Job drawing, mm, ordinate dimensions from the low corner. One solid piece. A direction names the side the tool comes from. Give positions to 0.01 mm unless a question says otherwise; leave off trailing zeros. Order: outer loops, then holes, each group sorted by start corner. A loop starts at its lowest first (then second) coordinate and runs counter-clockwise, first axis right, second up.
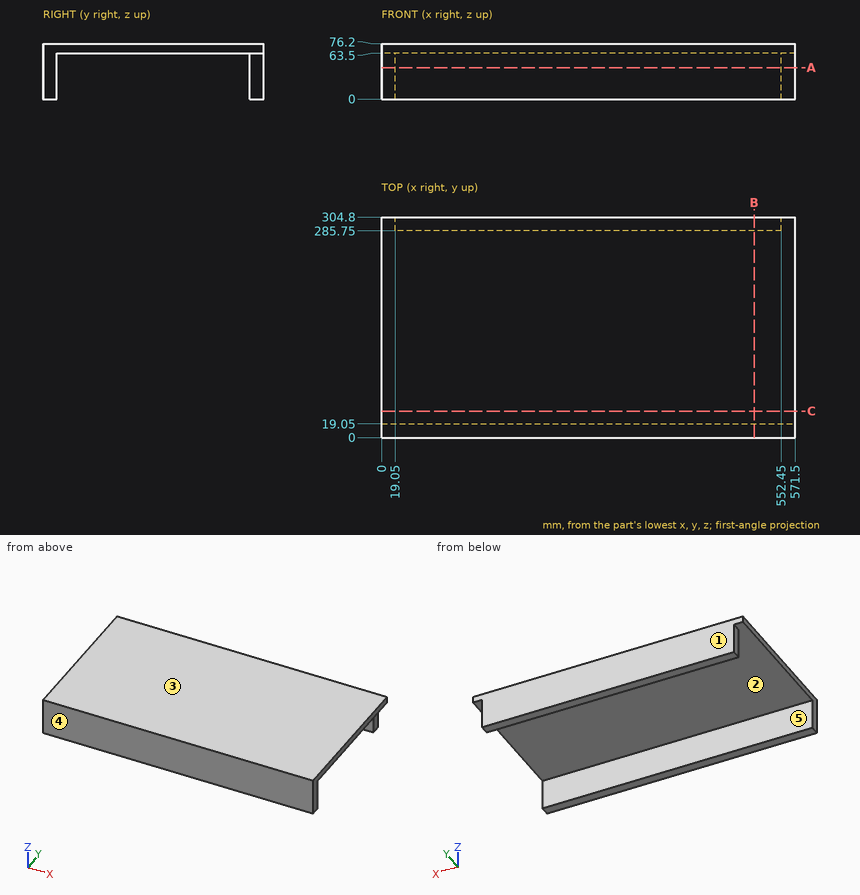
Item 1: Band-saw the part on C-C on y = 36.5. List the corners of the cut face in (x, z).
Item 2: Pull direction Y, two halves, no side cores. Call the marked faces 1, 2 and 3: released by +Y, released by -Y, zero draft, split by the parting line, or undercut.
Item 3: Drop flat-ended pins along their axis: P1, Ø21, axis at y = 298.5, z = 38, coming from the -X side; P2, Ø5.5, axis at y = 298.5, z = 43, coming from the +X side. Give the stop position or say it passes through.
Item 4: Drill centre lines: probe 1 along Y at (x, z) = (505.5, 8.5); probe 2 along Z at (x, y) = (119.5, 110.5). Where is each one in solid material? Low to high.
Item 5: Band-saw the part on A-A on z = 43.5. List the corners of the cut face in (x, y), plus the area to 3 significant figures.
Item 6: Which spindle directions (+Z, -Z, +X, -X, +Y, -Y) get a long thin tool onto all of the face, cutting with end or side? Do the marked faces 4 and 5. Say none if no direction does.
Item 7: Band-saw the part on B-B on x = 515. List the corners of the cut face in (y, z), plus the area to 3 significant figures.
Working result:
1. outline: (0, 63.5) - (571.5, 63.5) - (571.5, 76.2) - (0, 76.2) - close
2. face 1: released by +Y
2. face 2: undercut
2. face 3: zero draft
3. P1: stops at x = 19.05
3. P2: stops at x = 552.45
4. probe 1: y = 0 to 19.05, 285.75 to 304.8
4. probe 2: z = 63.5 to 76.2
5. outline: (0, 0) - (571.5, 0) - (571.5, 19.05) - (0, 19.05) - close; (19.05, 285.75) - (552.45, 285.75) - (552.45, 304.8) - (19.05, 304.8) - close
5. area: 21,000 mm2
6. face 4: +Z, -Z, +X, -X, -Y
6. face 5: -Z, +X, -X
7. outline: (0, 0) - (19.05, 0) - (19.05, 63.5) - (285.75, 63.5) - (285.75, 0) - (304.8, 0) - (304.8, 76.2) - (0, 76.2) - close
7. area: 6,290 mm2
